Input: part model. Units: mm. Frame: model coordinates. A direction names the side the tool comes from. Round coordinates to 2 decimals unless told otherwise and drop trailing zeros. Loops run counter-clockwise (first coordinate to the right, second up) from the corner with the lowest first, then second, coordinate; pieces in that order, holes last. Notation, with made-up numbers: (3, 40) -> (31, 40) arc R18 ccw to (31, 54) -> close; hole circle Ø2 at (82, 7). An arc over 180 degrees is marked (long way). Answer as a JSON object with one key per item and string values. Group by question number.
Item 1: Material intervals for line 1 (X direction, y = -11.75, z = -0.5); line 2 (X direction, y = 10.5, z = -2.8); line 3 (X direction, y = 2, z = -0.6), sorted ascending. Write a range as [from, to].
Item 2: Draft query along X for faces 1 (the flat face through (-8, -2, 0)), 2 (the flat face through (6, 0, -1)), 3 (the flat face through (35.018, 0, -1)). Return one class per face: released by +X, released by -X, zero draft, split by the parting line, or undercut.
Item 3: Section query C-C on z = -1.3. Return loops of the section in (x, y), and give its area (3 significant figures).
Item 4: Section query D-D on x = -19. Return loops of the section in (y, z).
Item 5: Section query B-B on x = 4. Return loops of the section in (y, z), and give its area (3 significant figures).
Item 6: Section query A-A on y = 0.75. Return loops of the section in (x, z).
Item 7: Set-up query: faces 4 (the flat face through (-31, 9.75, -1)), 5 (the flat face through (34, -12.5, -1)), 6 (the flat face through (-32.518, -11, -1)). Return all of +Z, -Z, +X, -X, +Y, -Y with unobstructed straight access to the full face (end or side cutting, diameter ignored); none if empty.
Item 8: Pin query (flat end, axial travel): pin 1 (1.5 mm diameter, centred on x = 31, z = -1, fed in from -Y); pin 2 (1.5 mm diameter, centred on x = -31, z = -1, fed in from +Y); pin 3 (1.5 mm diameter, centred on x = 23, z = -2, fed in from -Y). Return the tip coordinate at first contact, or that it passes through.
from build123d import *

# Parameters (mm, degrees)
AUFSATZ_LINEAR_AUSTRAGEN1_DEPTH      = 3
SCHNITT_LINEAR_AUSTRAGEN2_DEPTH      = 39.826708727
SCHNITT_LINEAR_AUSTRAGEN2_DEPTH_BACK = 39.826708727
SKIZZE5_W                            = 3.3
SKIZZE5_H                            = 1.1
SCHNITT_LINEAR_AUSTRAGEN3_DEPTH      = 10


with BuildPart() as part:
    # Skizze1 → Aufsatz-Linear austragen1 (new body)
    with BuildSketch(Plane.XY):
        with BuildLine():
            Line((-6, -11.25), (0, -11.25))
            Line((0, -11.25), (0, -16.5))
            ThreePointArc((0, -16.5), (-14.893915213, -15.49545091), (-29.518042644, -12.5))
            Line((-29.518042644, -12.5), (-29.518042644, -9.75))
            Line((-29.518042644, -9.75), (-32.518042644, -9.75))
            Line((-32.518042644, -9.75), (-32.518042644, -12.5))
            Line((-32.518042644, -12.5), (-35.018042644, -12.5))
            Line((-35.018042644, -12.5), (-35.018042644, 12.5))
            Line((-35.018042644, 12.5), (-32.518042644, 12.5))
            Line((-32.518042644, 12.5), (-32.518042644, 9.75))
            Line((-32.518042644, 9.75), (-29.518042644, 9.75))
            Line((-29.518042644, 9.75), (-29.518042644, 12.5))
            ThreePointArc((-29.518042644, 12.5), (-14.893915213, 15.49545091), (0, 16.5))
            Line((0, 16.5), (0, 11.25))
            Line((0, 11.25), (-6, 11.25))
            Line((-6, 11.25), (-6, -11.25))
        make_face()
    aufsatz_linear_austragen1 = extrude(amount=-AUFSATZ_LINEAR_AUSTRAGEN1_DEPTH)

    # Spiegeln1: Aufsatz-Linear austragen1 across plane
    add(aufsatz_linear_austragen1.mirror(Plane(origin=(0, 0, 0), x_dir=(0, 0, 1), z_dir=(1, 0, 0))))

    # Skizze2 → Schnitt-Linear austragen2 (cut, two sides: drawn at the far end of the back side and taken through both)
    with BuildSketch(Plane.XY.offset(-SCHNITT_LINEAR_AUSTRAGEN2_DEPTH_BACK)):
        Polygon((181.022901985, 12.5), (29.518042644, 12.5), (-29.518042644, 12.5), (-181.022901985, 12.5), (-181.022901985, 315.509718682), (181.022901985, 315.509718682), align=None)
    extrude(amount=SCHNITT_LINEAR_AUSTRAGEN2_DEPTH + SCHNITT_LINEAR_AUSTRAGEN2_DEPTH_BACK, mode=Mode.SUBTRACT)

    # Skizze5 → Schnitt-Linear austragen3 (cut)
    with BuildSketch(Plane.XY):
        with Locations((0, -11.8)):
            Rectangle(SKIZZE5_W, SKIZZE5_H)
    extrude(amount=-SCHNITT_LINEAR_AUSTRAGEN3_DEPTH, mode=Mode.SUBTRACT)


solid = part.part
Solved:
{
 "1": {"line 1": "[-35.02, -32.52], [-29.52, -1.65], [1.65, 29.52], [32.52, 35.02]", "line 2": "[-35.02, -32.52], [-29.52, -6], [6, 29.52], [32.52, 35.02]", "line 3": "[-35.02, -6], [6, 35.02]"},
 "2": {"face 1": "zero draft", "face 2": "undercut", "face 3": "released by +X"},
 "3": {"outline": "(-35.02, -12.5) -> (-32.52, -12.5) -> (-32.52, -9.75) -> (-29.52, -9.75) -> (-29.52, -12.5) arc R110.91 ccw to (29.52, -12.5) -> (29.52, -9.75) -> (32.52, -9.75) -> (32.52, -12.5) -> (35.02, -12.5) -> (35.02, 12.5) -> (32.52, 12.5) -> (32.52, 9.75) -> (29.52, 9.75) -> (29.52, 12.5) -> (-29.52, 12.5) -> (-29.52, 9.75) -> (-32.52, 9.75) -> (-32.52, 12.5) -> (-35.02, 12.5) -> close; hole (-6, -11.25) -> (-1.65, -11.25) -> (-1.65, -12.35) -> (1.65, -12.35) -> (1.65, -11.25) -> (6, -11.25) -> (6, 11.25) -> (-6, 11.25) -> close", "area": "1,600 mm²"},
 "4": {"outline": "(-14.86, -3) -> (12.5, -3) -> (12.5, 0) -> (-14.86, 0) -> close"},
 "5": {"outline": "(-16.43, -3) -> (-11.25, -3) -> (-11.25, 0) -> (-16.43, 0) -> close; (11.25, -3) -> (12.5, -3) -> (12.5, 0) -> (11.25, 0) -> close", "area": "19.3 mm²"},
 "6": {"outline": "(-35.02, -3) -> (-6, -3) -> (-6, 0) -> (-35.02, 0) -> close; (6, -3) -> (35.02, -3) -> (35.02, 0) -> (6, 0) -> close"},
 "7": {"face 4": "+Z, -Z, +Y", "face 5": "+Z, -Z, +X, -Y", "face 6": "+Z, -Z, -Y"},
 "8": {"pin 1": "y = -9.75", "pin 2": "y = 9.75", "pin 3": "y = -14.25"}
}
